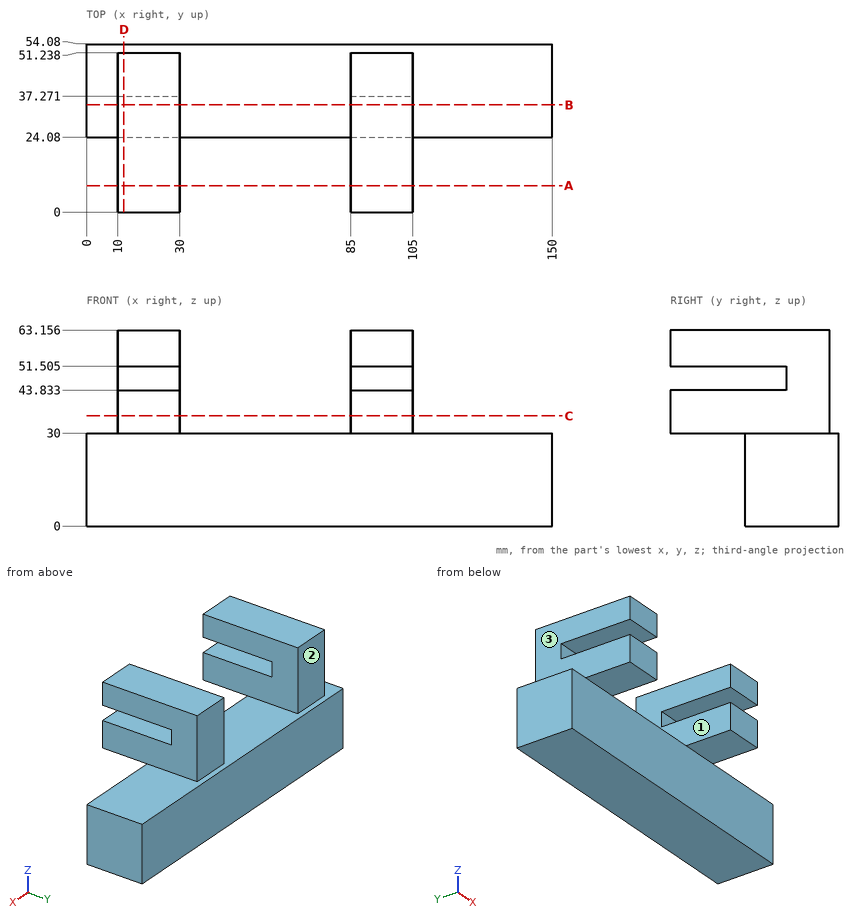
Geometry check sheet. Reference: drawing and pictorial views, mm from the part's lowest x, y, z. A direction names the side the tool comes from. Round coordinates to 2 decimals unless told otherwise and drop trailing zeros. Order: outer loops, then holes, each group sorted by start corner. A loop starts at its lowest first (then second) coordinate and runs counter-clockwise, first axis right, second up. Notation, with made-up numbers: (82.5, 23.5) -> (133.5, 23.5) arc R28 cw to (133.5, 60.5) -> close; hole circle Ø5 at (22, -17). An arc over 180 degrees is marked (long way). One line per item, written item: value. Start each with the question number.
Q1. Cross-section at A-A (y = 8.5). Record the boundary of the cut face in (x, z) (1 decimal).
Q2. Cross-section at C-C (z = 35.5). Record the boundary of the cut face in (x, y).
Q3. Set-up check for the marked faces 1, 2 and 3: record each of +Z, -Z, +X, -X, +Y, -Y from which the full face is reachable in a straight line by a thin tool's end or side.
Q4. Thickness scan on line 1 (X direction, y = 40.5, z = 46); line 2 (Z direction, x = 102, y = 13.5) (1 decimal); line 3 (Y direction, x = 61, z = 21.5). Record the ranges inside material, lowest first.
Q5. Cross-section at B-B (y = 34.5). Record the boundary of the cut face in (x, z) (1 decimal), and give its area (3 significant figures).
Q6. Gauge pin test, flat ends, axial feed: pin 1 Ø1 at (x, z) = (101, 46) entering from -Y; pin 2 Ø16 at (x, z) = (98.5, 52) entering from +Y; pin 3 Ø10 at (x, z) = (118.5, 31.5) entering from +Y; pin 4 Ø12 at (x, z) = (121.5, 24.5) entering from -Y. Record the tip position at first contact, or that the pin passes through.
Q7. Cross-section at D-D (x = 12). Record the boundary of the cut face in (y, z) (1 decimal).
Completed:
1. outline: (10, 30) -> (30, 30) -> (30, 43.8) -> (10, 43.8) -> close; (10, 51.5) -> (30, 51.5) -> (30, 63.2) -> (10, 63.2) -> close; (85, 30) -> (105, 30) -> (105, 43.8) -> (85, 43.8) -> close; (85, 51.5) -> (105, 51.5) -> (105, 63.2) -> (85, 63.2) -> close
2. outline: (10, 0) -> (30, 0) -> (30, 51.24) -> (10, 51.24) -> close; (85, 0) -> (105, 0) -> (105, 51.24) -> (85, 51.24) -> close
3. face 1: +Z, +Y, -Y
3. face 2: +Z, +X, -X, +Y
3. face 3: +Z, -X, +Y, -Y
4. line 1: x = 10 to 30, 85 to 105
4. line 2: z = 30 to 43.8, 51.5 to 63.2
4. line 3: y = 24.08 to 54.08
5. outline: (0, 0) -> (150, 0) -> (150, 30) -> (105, 30) -> (105, 43.8) -> (85, 43.8) -> (85, 30) -> (30, 30) -> (30, 43.8) -> (10, 43.8) -> (10, 30) -> (0, 30) -> close; (10, 51.5) -> (30, 51.5) -> (30, 63.2) -> (10, 63.2) -> close; (85, 51.5) -> (105, 51.5) -> (105, 63.2) -> (85, 63.2) -> close
5. area: 5,520 mm²
6. pin 1: stops at y = 37.27
6. pin 2: stops at y = 51.24
6. pin 3: stops at y = 54.08
6. pin 4: stops at y = 24.08
7. outline: (0, 30) -> (24.1, 30) -> (24.1, 0) -> (54.1, 0) -> (54.1, 30) -> (51.2, 30) -> (51.2, 63.2) -> (0, 63.2) -> (0, 51.5) -> (37.3, 51.5) -> (37.3, 43.8) -> (0, 43.8) -> close
